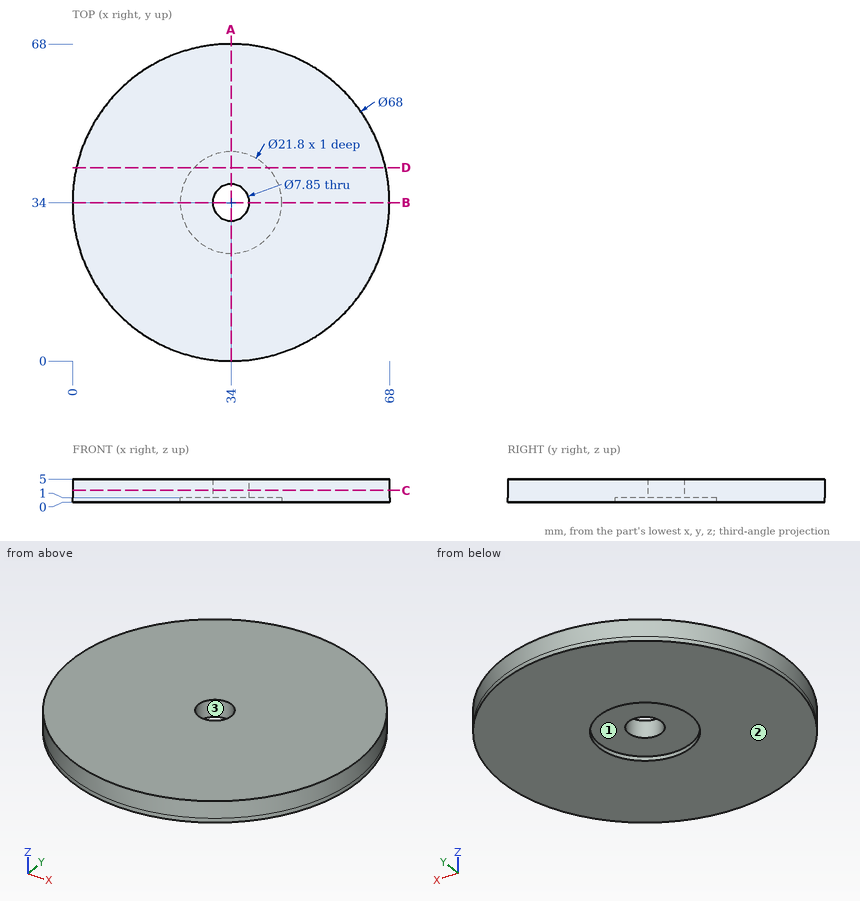
Geometry check sheet. Reference: drawing and pictorial views, mm from the part's lowest x, y, z. Give positions to 0.01 mm unless a question says otherwise; leave off trailing zeros. Order: outer loops, then holes, each group sorted by start corner. A loop starts at its lowest first (then second) coordinate and runs counter-clockwise, first axis right, second up. Notation, with made-up numbers: (-20.5, 75) - (1.5, 75) arc R36 cw to (1.5, 113) - close; hole circle Ø8 at (88, 59). An arc over 180 degrees is marked (long way). Answer as CSV lines item,"result".
1. Scan lines: probe 1 along Y at (x, z) = (34, 0.4); probe 2 along Y at (x, z) = (34, 3) (3 decimals); probe 3 along X at (y, z) = (37.5, 1.6). Record each from-to range of solid material in increasing order. Write a range as from..to.
Result sheet:
probe 1,"0..23.1, 44.9..68"
probe 2,"0..30.075, 37.925..68"
probe 3,"0.18..32.22, 35.78..67.82"
2. Section check D-D (y = 41.5). Record the boundary of the cut face in (x, z).
Result sheet:
outline,"(0.84, 0) - (26.09, 0) - (26.09, 1) - (41.91, 1) - (41.91, 0) - (67.16, 0) - (67.16, 5) - (0.84, 5) - close"
3. Go/stop test with flat-tipped pins: P1, Ø17.5, axis at x = 34, y = 34, coming from the -Z side; P2, Ø3, axis at y = 16, z = 1, coming from the +X side; P3, Ø6.5, axis at x = 34, y = 34, coming from the +Z side; P4, Ø1.5, axis at x = 48.5, z = 2.5, coming from the +Y side. Record where each tip stops, or that it passes through.
Result sheet:
P1,"z = 1"
P2,"x = 63.73"
P3,"through"
P4,"y = 65.1"
4. Section check A-A (x = 34). Record the boundary of the cut face in (y, z) (3 decimals), then the cut area to 3 significant figures.
Result sheet:
outline,"(0, 0) - (23.1, 0) - (23.1, 1) - (30.075, 1) - (30.075, 5) - (0, 5) - close; (37.925, 1) - (44.9, 1) - (44.9, 0) - (68, 0) - (68, 5) - (37.925, 5) - close"
area,"287 mm²"
5. Mould release check, pull along X, two halves, no side actions. Record for the marked faces 1, 2 and 3: released by +X, released by -X, zero draft, split by the parting line, or undercut.
Result sheet:
face 1,"undercut"
face 2,"zero draft"
face 3,"undercut"
6. Section check C-C (z = 2.55). Record the boundary of the cut face in (x, y) (3 decimals).
Result sheet:
outline,"circle Ø68 at (34, 34); hole circle Ø7.85 at (34, 34)"
